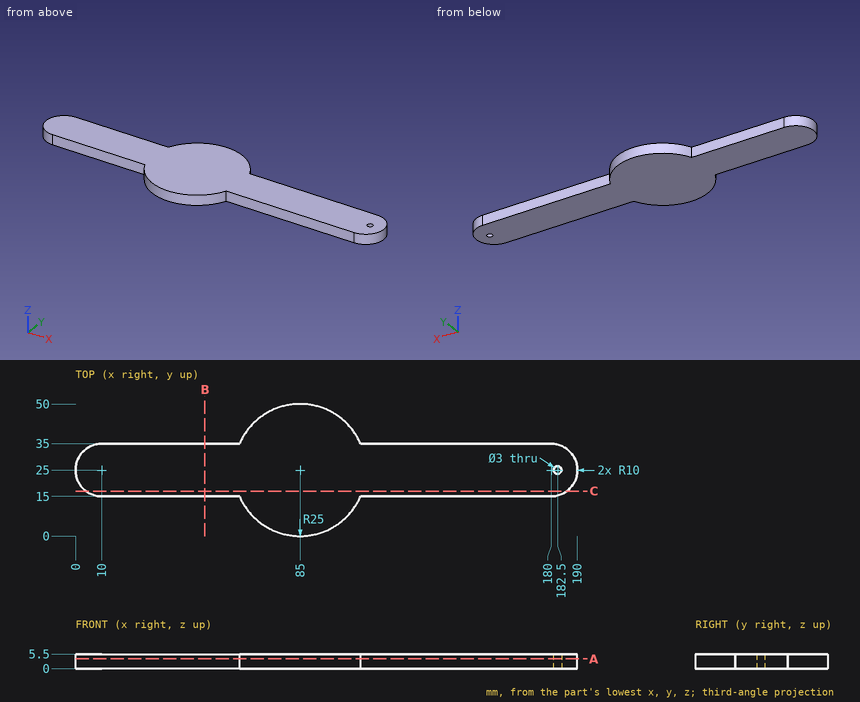
Input: dimensioned drawing with shaded views. Units: mm. Origin: part minimum x, y, z. Coordinates: 2 decimals unless noted, no trailing zeros. Order: outer loops, then holes, each group sorted by start corner. A loop starts at its lowest first (then second) coordinate and runs counter-clockwise, first axis right, second up.
Item 1: Section query A-A (z = 3.7). Output: boundary loops of the cut face in (x, y), then the cut area to 3 significant figures.
Answer:
outline: (10, 15) - (62.09, 15) arc R25 ccw to (107.91, 15) - (180, 15) arc R10 ccw to (180, 35) - (107.91, 35) arc R25 ccw to (62.09, 35) - (10, 35) arc R10 ccw to start; hole circle Ø3 at (182.5, 25)
area: 4,700 mm2
Item 2: Section query B-B (x = 49). Output: boundary loops of the cut face in (y, z).
Answer:
outline: (15, 0) - (35, 0) - (35, 5.5) - (15, 5.5) - close
Item 3: Section query C-C (y = 17). Output: boundary loops of the cut face in (x, z), then the cut area to 3 significant figures.
Answer:
outline: (4, 0) - (186, 0) - (186, 5.5) - (4, 5.5) - close
area: 1,000 mm2
Item 4: Contact query for flat-ended pins moving along their axis: P1, Ø1.6, axis at x = 161.5, z = 1.5, coming from the +Y side; P2, Ø3, axis at x = 76.5, z = 4.5, coming from the +Y side; P3, Ø1.5, axis at y = 29.5, z = 0.5, coming from the -X side. Output: stop coordinate, or through.
Answer:
P1: stops at y = 35
P2: stops at y = 49
P3: stops at x = 0.73
Item 5: Material intervals for line 1 along X through (y, z) = (25, 1.5); line 2 along Y through (x, z) = (26.5, 4.1); line 3 along Y through (x, z) = (182.5, 2.05), sorted ascending.
Answer:
line 1: x = 0 to 181, 184 to 190
line 2: y = 15 to 35
line 3: y = 15.32 to 23.5, 26.5 to 34.68
